Design review of the part built by this model. Coordinates are the model's own, in mm. Face numbers are marked on the shaded views. A direction names the side the tool comes from. Give positions to 0.01 mm unless a question says otherwise; leave off trailing zeros. Order: outer loops, then holes, each group sorted by start corner. A loop starts at its lowest first (then second) coordinate and runs counter-clockwise, first axis right, second up. Notation, with made-up numbers: (-15.5, 49.5) -> (1.5, 49.5) arc R29 cw to (1.5, 78.5) -> close; hole circle Ø10 at (3, 11.5). An arc over 180 degrees is marked (long way). Return JSON: item names as keys, results as strings.
Autodesk Inventor part; units mm, degrees
ref_plane "YZ Plane" through (0, 0, 0) normal (1, 0, 0) x (0, 1, 0)
ref_plane "XZ Plane" through (0, 0, 0) normal (0, 1, 0) x (-1, 0, 0)
ref_plane "XY Plane" through (0, 0, 0) normal (0, 0, 1) x (1, 0, 0)
sketch "Sketch1" plane through (0, 0, 0) normal (1, 0, 0) x (0, 1, 0)
  line L0 (0, 0) -> (15.5, 0)
  line L1 (15.5, 0) -> (15.5, -5)
  line L2 (15.5, -5) -> (0, -5)
  line L3 (0, -5) -> (0, 0)
  line L4 (15.5, 0) -> (10.5, 0)
  line L5 (10.5, 0) -> (10.5, 20.2)
  line L6 (10.5, 20.2) -> (15.5, 20.2)
  line L7 (15.5, 20.2) -> (15.5, 0)
  line L8 (15.5, 20.2) -> (0, 20.2)
  line L9 (0, 20.2) -> (0, 25.2)
  line L10 (0, 25.2) -> (15.5, 25.2)
  line L11 (15.5, 25.2) -> (15.5, 20.2)
  line L12 (2, 20.2) -> (0, 20.2)
  line L13 (0, 20.2) -> (0, 18.2)
  line L14 (0, 18.2) -> (2, 18.2)
  line L15 (2, 18.2) -> (2, 20.2)
  dimension "d0" = 5
  dimension "d2" = 5
  dimension "d3" = 20.2
  dimension "d4" = 5
  dimension "d16" = 10.5
  dimension "d23" = 2
  dimension "d24" = 2
extrude "Extrusion1" add sketch "Sketch1" along normal blind 8
sketch "Sketch2" plane through (0, 15.5, 25.2) normal (0, 1, 0) x (1, 0, 0)
  line L0 (0, 0) -> (8, 0) construction
  line L1 (3.9, 0) -> (3.9, 30.2) construction
  line L2 (0, 30.2) -> (8, 30.2) construction
  line L3 (0, 30.2) -> (0, 0) construction
  line L4 (0, 30.2) -> (0, 0) construction
  line L5 (0, 0) -> (8, 0) construction
  line L6 (8, 30.2) -> (8, 0) construction
  line L7 (0, 30.2) -> (8, 30.2) construction
  line L8 (3.9, 15.1) -> (1.5202, 15.1)
  point P0 (0, 25.2)
  point P1 (3.9, 10.1)
  point P2 (3.9, 20.1)
  dimension "d7" = 3.9
  dimension "d8" = 10
hole "Hole1" at (3.9, 15.5, 15.1) at (3.9, 15.5, 5.1) direction (0, -1, 0) diameter 4.3 depth 10 tip angle 118
sketch "Sketch4" plane through (0, 15.5, 25.2) normal (0, 1, 0) x (1, 0, 0)
  circle A0 centre (3.9, 10.1) radius 2.15
  circle A1 centre (3.9, 20.1) radius 2.15
  line L0 (0, 30.2) -> (0, 0)
  line L1 (0, 0) -> (8, 0)
  line L2 (8, 30.2) -> (8, 0)
  line L3 (0, 30.2) -> (8, 30.2)
  line L4 (0, 0) -> (8, 0)
  circle A2 centre (-0.5, 3.5) radius 2.6
  line L5 (2.1, 3.5) -> (2.1, 0)
  point P0 (0, 25.2)
  point P1 (0, 6.0515)
  point P2 (0, 0.9485)
  point P3 (2.1, 0)
  dimension "d19" = 5.2
  dimension "d20" = 0.5
  dimension "d63" = 3.5
extrude "Extrusion2" cut sketch "Sketch4" against normal through all contours A2 L0 | A2 L5 L1 L0 picked at (0.1891, 2.7097)
sketch "Sketch5" plane through (0, 0, 18.2) normal (0, -1, 0) x (1, 0, 0)
  arc A0 (0, 0.9485) -> (2.1, 3.5) centre (-0.5, 3.5) ccw
  line L0 (0, 0.9485) -> (0, 0)
  line L1 (0, 0) -> (8, 0)
  line L2 (8, 7) -> (8, 0)
  line L3 (2.1, 7) -> (8, 7)
  line L4 (2.1, 7) -> (2.1, 3.5)
  circle A1 centre (4, 4) radius 1.4
  point P0 (0, -18.2)
  point P1 (8, 3.5)
  dimension "d25" = 2.8
  dimension "d26" = 4
  dimension "d28" = 3
extrude "Extrusion3" add sketch "Sketch5" along normal blind 1.5 contours A1
sketch "Sketch6" plane through (0, 0, -5) normal (0, -1, 0) x (1, 0, 0)
  line L0 (0, 5) -> (0, 0)
  line L1 (0, 0) -> (8, 0)
  line L2 (8, 5) -> (8, 0)
  line L3 (0, 5) -> (8, 5)
  line L4 (0, 5) -> (8, 5)
  line L5 (0, 0) -> (0, 24.1485)
  line L6 (8, 0) -> (-7, 0)
  line L7 (-7, 0) -> (-7, -7.5)
  line L8 (-7, -7.5) -> (8, -7.5)
  line L9 (8, -7.5) -> (8, 0)
  dimension "d59" = 7.5
  dimension "d60" = 15
extrude "Extrusion4" add sketch "Sketch6" against normal blind 3 contours L1 L9 L8 L7 L6
fillet "Fillet1" radius 1.5 2 edges at (4, 3, -5) (0, 1.5, -5)
sketch "Sketch9" plane through (8, 0, 0) normal (1, 0, 0) x (0, 0, -1)
  line L0 (0, 0) -> (3.5, 0)
  circle A0 centre (0, 0) radius 4
  dimension "d64" = 8
extrude "Extrusion5" cut sketch "Sketch9" against normal blind 3
fillet "Fillet2" radius 2 2 edges at (5, 0, -2) (5, 2, 0)
sketch "Sketch10" plane through (-7, 0, -12.5) normal (0, -1, 0) x (1, 0, 0)
  line L0 (10, 12.5) -> (10, 8.5)
  line L1 (7, 12.5) -> (10, 12.5)
  line L2 (7, 12.5) -> (7, 9)
  arc A0 (5.5, 7.5) -> (7, 9) centre (5.5, 9) ccw
  line L3 (5.5, 7.5) -> (0, 7.5)
  line L4 (0, 7.5) -> (0, 0)
  line L5 (0, 0) -> (15, 0)
  line L6 (15, 8.5) -> (15, 0)
  line L7 (15, 8.5) -> (10, 8.5)
  line L8 (15, 0) -> (0, 0) construction
  line L9 (0, 7.5) -> (5.5, 7.5) construction
  point P0 (11, 3)
  point P1 (2.75, 3)
  dimension "d76" = 3
  dimension "d77" = 4
hole "Hole4" at (4, 0, -9.5) at (-4.25, 0, -9.5) direction (0, 1, 0) diameter 3.4 depth 10 tip angle 118
properties part number "Servo mount"
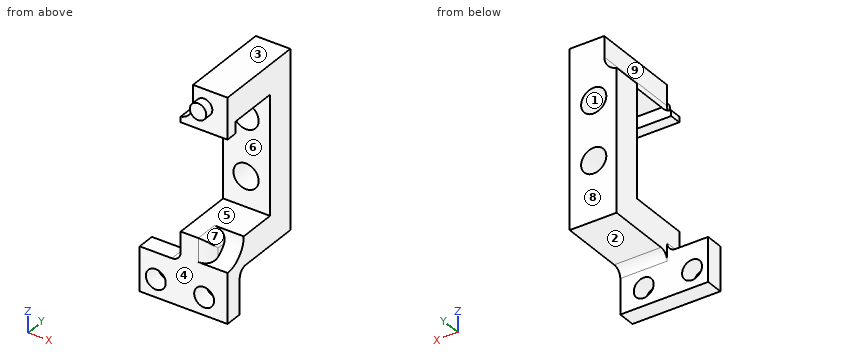
Item 1: Add section C-C (y = 0.5). Give the boundary of the cut face in (x, z).
Result set:
{"outline": "(-7, -12.5) -> (8, -12.5) -> (8, -3.97) -> (4.32, -3.97) -> (4.32, -0.5) arc R2 ccw to (3, 0) -> (0, 0) -> (0, -3.5) arc R1.5 cw to (-1.5, -5) -> (-7, -5) -> close; (0, 18.2) -> (8, 18.2) -> (8, 25.2) -> (2.1, 25.2) -> (2.1, 21.7) arc R2.6 cw to (0, 19.15) -> close; hole circle Ø3.4 at (-4.25, -9.5); hole circle Ø3.4 at (4, -9.5)"}
Item 2: Add section A-A (y = 7.25). Give the boundary of the cut face in (x, z).
Result set:
{"outline": "(0, -5) -> (8, -5) -> (8, 0) -> (0, 0) -> close; (1.62, 20.2) -> (8, 20.2) -> (8, 25.2) -> (2.1, 25.2) -> (2.1, 21.7) arc R2.6 cw to start"}
Item 3: Add section D-D (z = 15.1). Give the boundary of the cut face in (x, y), plus the area to 3 significant figures.
Result set:
{"outline": "(0, 10.5) -> (1.75, 10.5) -> (1.75, 15.5) -> (0, 15.5) -> close; (6.05, 10.5) -> (8, 10.5) -> (8, 15.5) -> (6.05, 15.5) -> close", "area": "18.5 mm^2"}
Item 4: For pin 1 (8 mm diameter, centred on x = -2.5, z = 20, fed in from -Y); pin 2 (1 mm diameter, centred on y = 9.5, z = 22.5, fed in from -X); pin 3 (4.5 mm diameter, centred on x = -2.5, z = -7, fed in from +Y), all flat-tipped, find the tip position at first contact; note any pin that passes through.
Result set:
{"pin 1": "stops at y = 0", "pin 2": "stops at x = 2.1", "pin 3": "stops at y = 3"}
Item 5: Add section B-B (x = -4.25). Give the boundary of the cut face in (y, z), plus the area to 3 significant figures.
Result set:
{"outline": "(0, -12.5) -> (3, -12.5) -> (3, -11.2) -> (0, -11.2) -> close; (0, -7.8) -> (3, -7.8) -> (3, -5) -> (0, -5) -> close", "area": "12.3 mm^2"}
Item 6: Machinability: for the marked faces 5, 6, 7, 8 and 9, which of the approach directions +Z, -Z, +X, -X, +Y, -Y give a long, thin tool a straight path to every point of the face, cutting with its end or side? Answer none if there is none.
Result set:
{"face 5": "+X, -X, -Y", "face 6": "+X, -X", "face 7": "+X, -Y", "face 8": "+Z, -Z, +X, -X, +Y", "face 9": "+Z, -X, +Y, -Y"}
Item 7: Wall thickness on L1, parallel to Z at x = 3.9, y = 13.15; L2, parallel to X at y = 1.95, z = -9.5; L3, parallel to Z at x = 5, y = 8.5: over which ranges is each line inside the solid? List them lowest first. Write a range as [from, to].
Result set:
{"L1": "z = [-5, 2.95], [7.25, 12.95], [17.25, 25.2]", "L2": "x = [-7, -5.95], [-2.55, 2.3], [5.7, 8]", "L3": "z = [-5, 0], [20.2, 25.2]"}
Item 8: Mouldability with a two-part tool opening along Z and no side actions: class the marked faces 1, 2, 3 and 4 as released by +Z, released by -Z, zero draft, split by the parting line, or undercut.
Result set:
{"face 1": "undercut", "face 2": "released by -Z", "face 3": "released by +Z", "face 4": "zero draft"}
